Geometry: final body of the model. Coordinates: model frame, mm. A direction names the side the tool comes from. Round coordinates to 2 decimals unless told otherwise and drop trailing zeros. Loops run counter-clockwise (first coordinate to the right, second up) from the corner with the lowest first, then second, coordinate; pieces in that order, holes last. Notation, with made-up numbers: (39, 48) -> (72, 48) arc R33 ccw to (72, 80) -> close; hole circle Ø1 at (-38.75, 5). An arc over 180 degrees is marked (long way). Answer in a Markdown table with one row per item.
```python
from build123d import *

# Parameters (mm, degrees)
SKETCH1_R           = 9.5
SKETCH1_R_2         = 2.25
BOSS_EXTRUDE1_DEPTH = 4
SKETCH2_R           = 9.5
CUT_EXTRUDE1_DEPTH  = 15.017845769


with BuildPart() as part:
    # Sketch1 → Boss-Extrude1 (new body)
    with BuildSketch(Plane.XY):
        Circle(SKETCH1_R)
        Circle(SKETCH1_R_2, mode=Mode.SUBTRACT)
    extrude(amount=BOSS_EXTRUDE1_DEPTH)

    # Sketch2 → Cut-Extrude1 (cut, through all)
    with BuildSketch(Plane.XY.offset(4)):
        Circle(SKETCH2_R)
        with BuildLine():
            ThreePointArc((5.362381822, 2.473224364), (6.518915118, 3.194006906), (7.223355975, 4.36056587))
            ThreePointArc((7.223355975, 4.36056587), (7.108458656, 4.54546167), (6.988829661, 4.727331828))
            ThreePointArc((6.988829661, 4.727331828), (5.634356921, 4.57733072), (4.4948488, 3.829923215))
            ThreePointArc((4.4948488, 3.829923215), (4.069180633, 4.279456337), (3.598788625, 4.681954506))
            ThreePointArc((3.598788625, 4.681954506), (4.287883651, 5.857643573), (4.369508071, 7.217950226))
            ThreePointArc((4.369508071, 7.217950226), (4.181846184, 7.32827188), (3.991400694, 7.433715542))
            ThreePointArc((3.991400694, 7.433715542), (2.861783635, 6.671441288), (2.200136889, 5.48008898))
            ThreePointArc((2.200136889, 5.48008898), (1.614317987, 5.680312931), (1.010756324, 5.818105294))
            ThreePointArc((1.010756324, 5.818105294), (1.074549714, 7.179364689), (0.514658525, 8.421789172))
            ThreePointArc((0.514658525, 8.421789172), (0.297223149, 8.432263317), (0.079589928, 8.437124611))
            ThreePointArc((0.079589928, 8.437124611), (-0.566389794, 7.237205057), (-0.598599868, 5.874832403))
            ThreePointArc((-0.598599868, 5.874832403), (-1.210365455, 5.779878288), (-1.80882807, 5.621398276))
            ThreePointArc((-1.80882807, 5.621398276), (-2.384950613, 6.856379876), (-3.458093086, 7.696297711))
            ThreePointArc((-3.458093086, 7.696297711), (-3.655490128, 7.604524849), (-3.85045393, 7.50769011))
            ThreePointArc((-3.85045393, 7.50769011), (-3.864810147, 6.145012365), (-3.26020461, 4.923722521))
            ThreePointArc((-3.26020461, 4.923722521), (-3.757768757, 4.555343184), (-4.214031752, 4.136896657))
            ThreePointArc((-4.214031752, 4.136896657), (-5.298087496, 4.962681062), (-6.638637245, 5.207677196))
            ThreePointArc((-6.638637245, 5.207677196), (-6.77077467, 5.034681382), (-6.898405196, 4.858334282))
            ThreePointArc((-6.898405196, 4.858334282), (-6.277849071, 3.645071395), (-5.174935765, 2.844647147))
            ThreePointArc((-5.174935765, 2.844647147), (-5.444312524, 2.287233855), (-5.653851544, 1.70468187))
            ThreePointArc((-5.653851544, 1.70468187), (-6.997496382, 1.932091823), (-8.298349616, 1.526040594))
            ThreePointArc((-8.298349616, 1.526040594), (-8.334956332, 1.311453085), (-8.366014967, 1.09599262))
            ThreePointArc((-8.366014967, 1.09599262), (-7.252708429, 0.310088497), (-5.904151501, 0.113897393))
            ThreePointArc((-5.904151501, 0.113897393), (-5.883629902, -0.504853187), (-5.798442084, -1.118054991))
            ThreePointArc((-5.798442084, -1.118054991), (-7.093863177, -1.541116368), (-8.057010096, -2.505193517))
            ThreePointArc((-8.057010096, -2.505193517), (-7.989699945, -2.712213309), (-7.91707153, -2.917427744))
            ThreePointArc((-7.91707153, -2.917427744), (-6.566059691, -3.095931939), (-5.280797281, -2.64294488))
            ThreePointArc((-5.280797281, -2.64294488), (-4.975078575, -3.181284447), (-4.614679421, -3.684658927))
            ThreePointArc((-4.614679421, -3.684658927), (-5.565111408, -4.661273372), (-5.969906661, -5.962517984))
            ThreePointArc((-5.969906661, -5.962517984), (-5.814099587, -6.11454432), (-5.654422416, -6.26250057))
            ThreePointArc((-5.654422416, -6.26250057), (-4.375205807, -5.792711678), (-3.447676044, -4.794320333))
            ThreePointArc((-3.447676044, -4.794320333), (-2.926796703, -5.12892178), (-2.373749315, -5.407151907))
            ThreePointArc((-2.373749315, -5.407151907), (-2.761459682, -6.713588821), (-2.515169554, -8.053901437))
            ThreePointArc((-2.515169554, -8.053901437), (-2.306559081, -8.116106915), (-2.096413271, -8.172909987))
            ThreePointArc((-2.096413271, -8.172909987), (-1.182045, -7.162450981), (-0.824733775, -5.847374775))
            ThreePointArc((-0.824733775, -5.847374775), (-0.208020978, -5.901584943), (0.410978151, -5.89093155))
            ThreePointArc((0.410978151, -5.89093155), (0.674809178, -7.227901978), (1.515762586, -8.300233131))
            ThreePointArc((1.515762586, -8.300233131), (1.729386313, -8.258367225), (1.941858891, -8.21100422))
            ThreePointArc((1.941858891, -8.21100422), (2.281908072, -6.891359081), (1.987145063, -5.560866125))
            ThreePointArc((1.987145063, -5.560866125), (2.558409847, -5.322266117), (3.101555477, -5.025169767))
            ThreePointArc((3.101555477, -5.025169767), (3.956487387, -6.086389898), (5.199451785, -6.645081443))
            ThreePointArc((5.199451785, -6.645081443), (5.369150144, -6.508735129), (5.535274583, -6.368056339))
            ThreePointArc((5.535274583, -6.368056339), (5.223103504, -5.041539866), (4.343792915, -4.000430061))
            ThreePointArc((4.343792915, -4.000430061), (4.738739807, -3.523680264), (5.08160382, -3.008202151))
            ThreePointArc((5.08160382, -3.008202151), (6.331782017, -3.550559241), (7.69200924, -3.467621679))
            ThreePointArc((7.69200924, -3.467621679), (7.778906383, -3.268030253), (7.860625575, -3.066263495))
            ThreePointArc((7.860625575, -3.066263495), (6.967748869, -2.036764624), (5.705330158, -1.523543681))
            ThreePointArc((5.705330158, -1.523543681), (5.833481586, -0.917861728), (5.897517968, -0.302091675))
            ThreePointArc((5.897517968, -0.302091675), (7.256541693, -0.201338251), (8.422420077, 0.504228423))
            ThreePointArc((8.422420077, 0.504228423), (8.406608915, 0.72134097), (8.385201978, 0.937973363))
            ThreePointArc((8.385201978, 0.937973363), (7.116166938, 1.434608847), (5.759845019, 1.302368196))
            ThreePointArc((5.759845019, 1.302368196), (5.591843034, 1.898227869), (5.362381822, 2.473224364))
        make_face(mode=Mode.SUBTRACT)
    extrude(amount=-CUT_EXTRUDE1_DEPTH, mode=Mode.SUBTRACT)


solid = part.part
```
Item 1: Ray query, L1, parallel to Y at x = 6, z = 2.65; L2, parallel to X at y = -1, z = 3.1; L3, parallel to Y at x = 0, z = 1.4. Return the intervals inside material, ascending.
Ans:
| item | result |
|---|---|
| L1 | -3.47 to -1.58, -0.32 to 1.37, 2.78 to 4.68 |
| L2 | -5.82 to -2.02, 2.02 to 5.82 |
| L3 | -5.91 to -2.25, 2.25 to 8.34 |
Item 2: Set-up query: faces 4 (the cylindrical face through (4.734, -3.531, 2.028)), 5 (the cylindrical face through (2.875, 6.686, 2.028)), 6 (the cylindrical face through (-1.19, -7.18, 2.03)). Return all of +Z, -Z, +X, -X, +Y, -Y with unobstructed straight access to the full face (end or side cutting, diameter ignored); none if empty.
Ans:
| item | result |
|---|---|
| face 4 | +Z, -Z |
| face 5 | +Z, -Z, +Y |
| face 6 | +Z, -Z, -Y |
Item 3: Mould query, pull axis X, two halves, no side actions, for faces 1 (the flat face through (2, -2, 4)), 2 (the cylindrical face through (-2.76, -6.69, 2.03)), 3 (the cylindrical face through (0.667, -7.21, 2.028)). Classes: released by +X, released by -X, zero draft, split by the parting line, or undercut.
Ans:
| item | result |
|---|---|
| face 1 | zero draft |
| face 2 | undercut |
| face 3 | undercut |
Item 4: Section query A-A, the plane x = -1.5. Output: boundary loops of the cut face in (y, z), and give its area (3 significant figures).
Ans:
| item | result |
|---|---|
| outline | (-7.63, 0) -> (-1.68, 0) -> (-1.68, 4) -> (-7.63, 4) -> close; (1.68, 0) -> (5.71, 0) -> (5.71, 4) -> (1.68, 4) -> close |
| area | 39.9 mm2 |
Item 5: Section query B-B, the plane y = 3.5. Output: boundary loops of the cut face in (x, z).
Ans:
| item | result |
|---|---|
| outline | (-6.14, 0) -> (6.78, 0) -> (6.78, 4) -> (-6.14, 4) -> close |
Item 6: First-contact query: P1, Ø3, axis at x = 2, y = 5, coming from the -Z side; P2, Ø2, axis at x = -6.5, z = 3, coming from the +Y side; P3, Ø1, axis at x = 2, y = 6.5, coming from the -Z side. Flat tips, straight axial feed; report the tip coordinate or a pass-through.
Ans:
| item | result |
|---|---|
| P1 | z = 0 |
| P2 | y = 5.21 |
| P3 | through |
